Build history of the part. All positions in model axes, mm. Face numbers are marked on the shaded views. A direction names the side the tool comes from. Round coordinates to 2 decimals unless told otherwise and drop trailing zeros. Write each loop counter-clockwise with the first axis right and the second up, starting at its lowest first coordinate (ties: lowest second). Pieces come first, ordered by that corner, then holes.
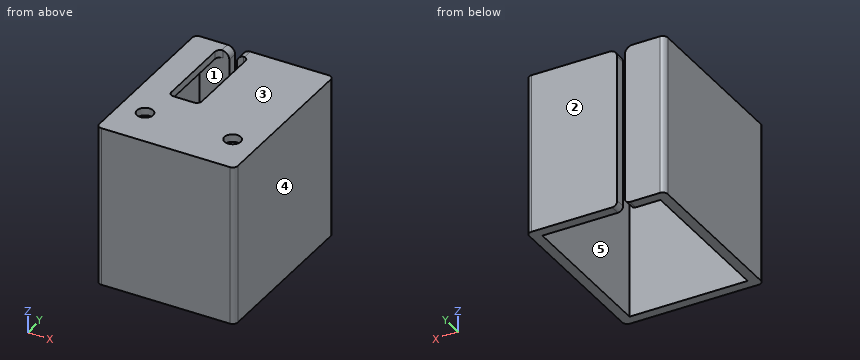
from build123d import *

# Parameters (mm, degrees)
SKETCH1_W           = 27.2
SKETCH1_H           = 34
SKETCH1_W_2         = 23.2
SKETCH1_H_2         = 30
BOSS_EXTRUDE1_DEPTH = 30
SKETCH2_W           = 27.2
SKETCH2_H           = 34
BOSS_EXTRUDE2_DEPTH = 1.5
SKETCH3_W           = 6
SKETCH3_H           = 17
SKETCH3_R           = 1.6
CUT_EXTRUDE1_DEPTH  = 31.5
FILLET1_R           = 1
SKETCH4_W           = 1.5
SKETCH4_H           = 2
CUT_EXTRUDE2_DEPTH  = 31.5
FILLET2_R           = 1
FILLET3_R           = 1.5


with BuildPart() as part:
    # Sketch1 → Boss-Extrude1 (new body)
    with BuildSketch(Plane.XY):
        Rectangle(SKETCH1_W, SKETCH1_H)
        Rectangle(SKETCH1_W_2, SKETCH1_H_2, mode=Mode.SUBTRACT)
    extrude(amount=BOSS_EXTRUDE1_DEPTH)

    # Sketch2 → Boss-Extrude2 (add)
    with BuildSketch(Plane.XY.offset(30)):
        Rectangle(SKETCH2_W, SKETCH2_H)
    extrude(amount=BOSS_EXTRUDE2_DEPTH)

    # Sketch3 → Cut-Extrude1 (cut)
    with BuildSketch(Plane.XY.offset(31.5)):
        with Locations((-5, 6.5)):
            Rectangle(SKETCH3_W, SKETCH3_H)
        with Locations((-8.6, -9)):
            Circle(SKETCH3_R)
        with Locations((8.6, -9)):
            Circle(SKETCH3_R)
    extrude(amount=-CUT_EXTRUDE1_DEPTH, mode=Mode.SUBTRACT)

    # Fillet1
    fillet1_edges = [part.edges().sort_by_distance(p)[0] for p in [
        (-8, -2, 30.75),
        (-2, -2, 30.75),
        (-2, 15, 30.75),
        (-8, 15, 30.75),
        (-13.6, 17, 15.75),
        (13.6, 17, 15.75),
        (13.6, -17, 15.75),
        (-13.6, -17, 15.75),
    ]]
    fillet(fillet1_edges, radius=FILLET1_R)

    # Sketch4 → Cut-Extrude2 (cut)
    with BuildSketch(Plane.XY.offset(31.5)):
        with Locations((-5, 16)):
            Rectangle(SKETCH4_W, SKETCH4_H)
    extrude(amount=-CUT_EXTRUDE2_DEPTH, mode=Mode.SUBTRACT)

    # Fillet2
    fillet2_edges = [part.edges().sort_by_distance(p)[0] for p in [
        (-4.25, 16, 0),
        (-5.75, 16, 0),
    ]]
    fillet(fillet2_edges, radius=FILLET2_R)

    # Fillet3
    fillet3_edges = [part.edges().sort_by_distance(p)[0] for p in [
        (-5.75, 16, 31.5),
        (-4.25, 16, 31.5),
    ]]
    fillet(fillet3_edges, radius=FILLET3_R)


solid = part.part
1) Wall check: L1, parallel to X at y = -12.5, z = 7.5; L2, parallel to Y at x = -9.75, z = 15; L3, parallel to Y at x = 8.6, z = 30.8. Give the ranges that are in metal, low to high.
Results:
L1: x = -13.6 to -11.6, 11.6 to 13.6
L2: y = -17 to -15, 15 to 17
L3: y = -17 to -10.6, -7.4 to 17
2) Mould opens along X. For the marked faces 3, 4 and 5 say: released by +X, released by -X, zero draft, split by the parting line, or undercut.
Results:
face 3: zero draft
face 4: released by +X
face 5: undercut
3) Slice it at B-B (y = -9). Write the cut outline in (x, z).
Results:
outline: (-13.6, 0) - (-11.6, 0) - (-11.6, 30) - (-10.2, 30) - (-10.2, 31.5) - (-13.6, 31.5) - close; (-7, 30) - (7, 30) - (7, 31.5) - (-7, 31.5) - close; (10.2, 30) - (11.6, 30) - (11.6, 0) - (13.6, 0) - (13.6, 31.5) - (10.2, 31.5) - close
4) Slice it at C-C (y = 5.5). Write the cut outline in (x, z), plus the area to 3 significant figures.
Results:
outline: (-13.6, 0) - (-11.6, 0) - (-11.6, 30) - (-8, 30) - (-8, 31.5) - (-13.6, 31.5) - close; (-2, 30) - (11.6, 30) - (11.6, 0) - (13.6, 0) - (13.6, 31.5) - (-2, 31.5) - close
area: 152 mm2
5) Slice it at D-D (z = 26.5). Write the cut outline in (x, y), plus the area to 3 significant figures.
Results:
outline: (-13.6, -16) arc R1 ccw to (-12.6, -17) - (12.6, -17) arc R1 ccw to (13.6, -16) - (13.6, 16) arc R1 ccw to (12.6, 17) - (-4.25, 17) - (-4.25, 15) - (11.6, 15) - (11.6, -15) - (-11.6, -15) - (-11.6, 15) - (-5.75, 15) - (-5.75, 17) - (-12.6, 17) arc R1 ccw to (-13.6, 16) - close
area: 225 mm2
6) Pin check, flat tips, straight feed: pin 1 Ø7 at (x, y) = (4.5, 0.5) entering from -Z; pin 2 Ø5 at (x, y) = (-8.6, -9) entering from +Z. Stop position of each tip, or through.
Results:
pin 1: stops at z = 30
pin 2: stops at z = 31.5
7) Slice it at A-A (x = -8.6). Write the cut outline in (y, z).
Results:
outline: (-17, 0) - (-15, 0) - (-15, 30) - (-10.6, 30) - (-10.6, 31.5) - (-17, 31.5) - close; (-7.4, 30) - (15, 30) - (15, 0) - (17, 0) - (17, 31.5) - (-7.4, 31.5) - close
8) Which spindle directions (+Z, -Z, +X, -X, +Y, -Y) get a long thin tool onto all of the face, cutting with end or side? Do the marked faces 1 and 2. Say none if no direction does.
Results:
face 1: -Z
face 2: +Z, -Z, +X, -X, +Y
